Source: CAD feature listing. Evaluate the final solid. Frame: model axes, mm. A direction names the side the tool comes from. Give positions to 0.01 mm unless a question says otherwise; leave off trailing zeros. Loops run counter-clockwise (first coordinate to the right, second up) from the corner with the lowest first, then second, coordinate; pieces in that order, holes last. Notation, with made-up numbers: (84.5, 47.25) -> (134.5, 47.25) arc R24 cw to (134.5, 63.25) -> close; hole circle Ø8 at (56.5, 1). An arc over 180 degrees is marked (long way). Answer as a JSON object with one key per item and string values. Group by question number.
from build123d import *

# Parameters (mm, degrees)
SKETCH1_W                               = 25
SKETCH1_H                               = 100
BOSS_EXTRUDE1_DEPTH                     = 10
CBORE_FOR_M5_HEX_HEAD_BOLT1_D           = 5.8
CBORE_FOR_M5_HEX_HEAD_BOLT1_CBORE_D     = 12.24
CBORE_FOR_M5_HEX_HEAD_BOLT1_CBORE_DEPTH = 3.58
FILLET1_R                               = 4


with BuildPart() as part:
    # Sketch1 → Boss-Extrude1 (new body)
    with BuildSketch(Plane(origin=(0, 0, 0), x_dir=(1, 0, 0), z_dir=(0, 1, 0))):
        with Locations((12.5, 50)):
            Rectangle(SKETCH1_W, SKETCH1_H)
    extrude(amount=BOSS_EXTRUDE1_DEPTH)

    # CBORE for M5 Hex Head Bolt1 (through all)
    with Locations(Plane(origin=(0, 10, 0), x_dir=(1, 0, 0), z_dir=(0, 1, 0))):
        with Locations((12.5, 67)):
            CounterBoreHole(CBORE_FOR_M5_HEX_HEAD_BOLT1_D / 2, CBORE_FOR_M5_HEX_HEAD_BOLT1_CBORE_D / 2, CBORE_FOR_M5_HEX_HEAD_BOLT1_CBORE_DEPTH)

    # Fillet1
    fillet1_edges = [part.edges().sort_by_distance(p)[0] for p in [
        (0, 5, -100),
        (25, 5, -100),
        (25, 5, 0),
        (0, 5, 0),
    ]]
    fillet(fillet1_edges, radius=FILLET1_R)


solid = part.part
(1) Mould query, pull axis Z, two halves, no side actions, for faces 1 (the face through (14, 6.42, -64)), 2 (the face through (1.141, 5.07, -1.203)), 3 (the face through (1.141, 5.07, -98.797)). Classes: pulls with the +Z half, pulls with the -Z half, needs draft (parallel to the pull), parting line crosses it, or undercut.
(2) Section query A-A on x = 12.5. Return the cut outline in (y, z).
(3) First-contact query: pin 1 (3.5 mm diameter, centred on x = 15, z = -67.5, fed in from +Y). Flat tip, straight axial feed; report the tip coordinate or a pass-through.
(4) Section query B-B on z = -67. Return the cut outline in (x, y).
(5) Material intervals for line 1 (X direction, y = 8.35, z = -67); line 2 (Z direction, x = 12.25, y = 5.25); line 3 (X direction, y = 3.5, z = -67), sorted ascending. Write a range as from..to.
(6) Section query C-C on y = 9. Return the cut outline in (x, z), plus the area to 3 significant figures.
(7) Access query for faces 4 (the face through (11.703, 8.235, -73.068)), 5 (the face through (12, 0, -51)). Directions: +Z, -Z, +X, -X, +Y, -Y. A direction counts if a zero-diameter tool reaches every point of the face in a straight line with its end or side. Return the directions, or none.
Result:
{
 "1": {"face 1": "undercut", "face 2": "pulls with the +Z half", "face 3": "pulls with the -Z half"},
 "2": {"outline": "(0, -100) -> (10, -100) -> (10, -73.12) -> (6.42, -73.12) -> (6.42, -69.9) -> (0, -69.9) -> close; (0, -64.1) -> (6.42, -64.1) -> (6.42, -60.88) -> (10, -60.88) -> (10, 0) -> (0, 0) -> close"},
 "3": {"pin 1": "y = 6.42"},
 "4": {"outline": "(0, 0) -> (9.6, 0) -> (9.6, 6.42) -> (6.38, 6.42) -> (6.38, 10) -> (0, 10) -> close; (15.4, 0) -> (25, 0) -> (25, 10) -> (18.62, 10) -> (18.62, 6.42) -> (15.4, 6.42) -> close"},
 "5": {"line 1": "0..6.38, 18.62..25", "line 2": "-100..-69.89, -64.11..0", "line 3": "0..9.6, 15.4..25"},
 "6": {"outline": "(0, -96) arc R4 ccw to (4, -100) -> (21, -100) arc R4 ccw to (25, -96) -> (25, -4) arc R4 ccw to (21, 0) -> (4, 0) arc R4 ccw to (0, -4) -> close; hole circle Ø12.24 at (12.5, -67)", "area": "2,370 mm²"},
 "7": {"face 4": "+Y", "face 5": "+Z, -Z, +X, -X, -Y"}
}
